```python
from build123d import *

# Parameters (mm, degrees)
ESQUISSE1_W             = 15.5
ESQUISSE1_H             = 2
EXTRU_MINCE1_DEPTH      = 84
ESQUISSE2_R             = 1.5
ENL_V_MAT_EXTRU_1_DEPTH = 86.441500455
CONG_1_R                = 5


with BuildPart() as part:
    # Esquisse1 → Extru.-Mince1 (new body)
    with BuildSketch(Plane.XY):
        with Locations((7.75, 1)):
            Rectangle(ESQUISSE1_W, ESQUISSE1_H)
    extrude(amount=EXTRU_MINCE1_DEPTH)

    # Esquisse2 → Enlèv. mat.-Extru.1 (cut, through all)
    with BuildSketch(Plane(origin=(0, 2, 0), x_dir=(1, 0, 0), z_dir=(0, 1, 0))):
        with Locations(Location((7.75, -24, 0), (0, 0, 270))):
            Circle(ESQUISSE2_R)
        with Locations(Location((7.75, -7, 0), (0, 0, 270))):
            Circle(ESQUISSE2_R)
        with Locations(Location((7.75, -77, 0), (0, 0, 90))):
            Circle(ESQUISSE2_R)
        with Locations(Location((7.75, -60, 0), (0, 0, 90))):
            Circle(ESQUISSE2_R)
    extrude(amount=-ENL_V_MAT_EXTRU_1_DEPTH, mode=Mode.SUBTRACT)

    # Congé1
    cong_1_edges = [part.edges().sort_by_distance(p)[0] for p in [
        (0, 1, 84),
        (0, 1, 0),
        (15.5, 1, 0),
        (15.5, 1, 84),
    ]]
    fillet(cong_1_edges, radius=CONG_1_R)


solid = part.part
```
Model file for the job. Use its own axes, mm. Coordinates: 2 decimals unless noted, no trailing zeros. Write each loop counter-clockwise with the first axis right and the second up, starting at its lowest first coordinate (ties: lowest second). Pieces come first, ordered by that corner, then holes. Notation, with made-up numbers: (50.5, 41) - (74.5, 41) arc R8 ccw to (74.5, 53) - close; hole circle Ø7 at (7.5, 3). An arc over 180 degrees is marked (long way). Use a Markdown table: item, result. Add a question column.
Item 1: Band-saw the part on D-D, the plane z = 7.5. Write the cut outline in (x, y).
Item 2: Drill centre lines: line 1 along X through (y, z) = (1.55, 7); line 2 along X through (y, z) = (1.3, 6); line 3 along Z through (x, y) = (14.5, 1.4). Where is each one in solid material? Low to high.
Item 3: Band-saw the part on C-C, the plane y = 1.7. Write the cut outline in (x, z), and give its area (3 significant figures).
Item 4: Band-saw the part on B-B, the plane z = 24. Write the cut outline in (x, y), and give its area (3 significant figures).
Item 5: Band-saw the part on A-A, the plane x = 7.75. Write the cut outline in (y, z), and give its area (3 significant figures).
Item 6: Two-plate mould, pull along X, no slides. Class faces 1 (the face through (8.325, 1.014, 75.614)), 2 (the face through (1, 1, 82)), 3 (the face through (8, 1, 0)): pulls with the +X half, pulls with the -X half, needs draft (parallel to the pull), parting line crosses it, or undercut.
A:
| question | item | result |
|---|---|---|
| 1 | outline | (0, 0) - (6.34, 0) - (6.34, 2) - (0, 2) - close; (9.16, 0) - (15.5, 0) - (15.5, 2) - (9.16, 2) - close |
| 2 | line 1 | x = 0 to 6.25, 9.25 to 15.5 |
| 2 | line 2 | x = 0 to 6.63, 8.87 to 15.5 |
| 2 | line 3 | z = 2 to 82 |
| 3 | outline | (0, 5) arc R5 ccw to (5, 0) - (10.5, 0) arc R5 ccw to (15.5, 5) - (15.5, 79) arc R5 ccw to (10.5, 84) - (5, 84) arc R5 ccw to (0, 79) - close; hole circle Ø3 at (7.75, 7); hole circle Ø3 at (7.75, 24); hole circle Ø3 at (7.75, 60); hole circle Ø3 at (7.75, 77) |
| 3 | area | 1,250 mm² |
| 4 | outline | (0, 0) - (6.25, 0) - (6.25, 2) - (0, 2) - close; (9.25, 0) - (15.5, 0) - (15.5, 2) - (9.25, 2) - close |
| 4 | area | 25.0 mm² |
| 5 | outline | (0, 0) - (2, 0) - (2, 5.5) - (0, 5.5) - close; (0, 8.5) - (2, 8.5) - (2, 22.5) - (0, 22.5) - close; (0, 25.5) - (2, 25.5) - (2, 58.5) - (0, 58.5) - close; (0, 61.5) - (2, 61.5) - (2, 75.5) - (0, 75.5) - close; (0, 78.5) - (2, 78.5) - (2, 84) - (0, 84) - close |
| 5 | area | 144 mm² |
| 6 | face 1 | undercut |
| 6 | face 2 | pulls with the -X half |
| 6 | face 3 | needs draft |
